```python
from build123d import *

# Parameters (mm, degrees)
SKETCH1_W           = 25.5
SKETCH1_H           = 5.5
BOSS_EXTRUDE1_DEPTH = 5
CUT_EXTRUDE1_DEPTH  = 10
SKETCH5_W           = 60
SKETCH5_H           = 5
BOSS_EXTRUDE2_DEPTH = 5
SKETCH6_W           = 20.4
SKETCH6_H           = 5
CUT_EXTRUDE2_DEPTH  = 10


with BuildPart() as part:
    # Sketch1 → Boss-Extrude1 (new body)
    with BuildSketch(Plane.XY):
        Polygon((-155, 151.5), (-155, 146.5), (5, 146.5), (5, 151.5), (25, 151.5), (25, -8.5), (-170, -8.5), (-170, 17.5), (-150, 17.5), (-150, 22.5), (-170, 22.5), (-170, 41), (-170, 41.4), (-163.2, 41.4), (-163.2, 40), (-160, 40), (-160, 41.4), (-153, 41.4), (-153, 45.6), (-160, 45.6), (-160, 47), (-163.2, 47), (-163.2, 45.6), (-170, 45.6), (-170, 46), (-170, 64.5), (-150, 64.5), (-150, 69.5), (-170, 69.5), (-170, 88.4), (-163.2, 88.4), (-163.2, 87), (-160, 87), (-160, 88.4), (-153, 88.4), (-153, 92.6), (-160, 92.6), (-160, 94), (-163.2, 94), (-163.2, 92.6), (-170, 92.6), (-170, 111.5), (-150, 111.5), (-150, 116.5), (-170, 116.5), (-170, 146.5), (-175, 146.5), (-175, 151.5), align=None)
        with Locations((-58.25, 13.75)):
            Rectangle(SKETCH1_W, SKETCH1_H, mode=Mode.SUBTRACT)
        with Locations((-12.75, 2.75)):
            Rectangle(SKETCH1_W, SKETCH1_H, mode=Mode.SUBTRACT)
        with Locations((-58.25, 2.75)):
            Rectangle(SKETCH1_W, SKETCH1_H, mode=Mode.SUBTRACT)
        with Locations((-12.75, 13.75)):
            Rectangle(SKETCH1_W, SKETCH1_H, mode=Mode.SUBTRACT)
        with Locations((-12.75, 26.25)):
            Rectangle(SKETCH1_W, SKETCH1_H, mode=Mode.SUBTRACT)
        with Locations((-58.25, 26.25)):
            Rectangle(SKETCH1_W, SKETCH1_H, mode=Mode.SUBTRACT)
        with Locations((-58.25, 37.25)):
            Rectangle(SKETCH1_W, SKETCH1_H, mode=Mode.SUBTRACT)
        with Locations((-12.75, 37.25)):
            Rectangle(SKETCH1_W, SKETCH1_H, mode=Mode.SUBTRACT)
        with Locations((-12.75, 49.75)):
            Rectangle(SKETCH1_W, SKETCH1_H, mode=Mode.SUBTRACT)
        with Locations((-58.25, 49.75)):
            Rectangle(SKETCH1_W, SKETCH1_H, mode=Mode.SUBTRACT)
        with Locations((-58.25, 60.75)):
            Rectangle(SKETCH1_W, SKETCH1_H, mode=Mode.SUBTRACT)
        with Locations((-12.75, 60.75)):
            Rectangle(SKETCH1_W, SKETCH1_H, mode=Mode.SUBTRACT)
        with Locations((-12.75, 73.25)):
            Rectangle(SKETCH1_W, SKETCH1_H, mode=Mode.SUBTRACT)
        with Locations((-58.25, 73.25)):
            Rectangle(SKETCH1_W, SKETCH1_H, mode=Mode.SUBTRACT)
        with Locations((-58.25, 84.25)):
            Rectangle(SKETCH1_W, SKETCH1_H, mode=Mode.SUBTRACT)
        with Locations((-12.75, 84.25)):
            Rectangle(SKETCH1_W, SKETCH1_H, mode=Mode.SUBTRACT)
        with Locations((-12.75, 96.75)):
            Rectangle(SKETCH1_W, SKETCH1_H, mode=Mode.SUBTRACT)
        with Locations((-58.25, 96.75)):
            Rectangle(SKETCH1_W, SKETCH1_H, mode=Mode.SUBTRACT)
        with Locations((-58.25, 107.75)):
            Rectangle(SKETCH1_W, SKETCH1_H, mode=Mode.SUBTRACT)
        with Locations((-12.75, 107.75)):
            Rectangle(SKETCH1_W, SKETCH1_H, mode=Mode.SUBTRACT)
        with Locations((-12.75, 120.25)):
            Rectangle(SKETCH1_W, SKETCH1_H, mode=Mode.SUBTRACT)
        with Locations((-58.25, 120.25)):
            Rectangle(SKETCH1_W, SKETCH1_H, mode=Mode.SUBTRACT)
        with Locations((-58.25, 131.25)):
            Rectangle(SKETCH1_W, SKETCH1_H, mode=Mode.SUBTRACT)
        with Locations((-12.75, 131.25)):
            Rectangle(SKETCH1_W, SKETCH1_H, mode=Mode.SUBTRACT)
    extrude(amount=BOSS_EXTRUDE1_DEPTH)

    # Sketch4 → Cut-Extrude1 (cut)
    with BuildSketch(Plane.XY.offset(5)):
        Polygon((-37.8, 129.5), (-37.8, 136.5), (-39.2, 136.5), (-39.2, 139.7), (-37.8, 139.7), (-37.8, 146.5), (-33.6, 146.5), (-33.6, 139.7), (-32.2, 139.7), (-32.2, 136.5), (-33.6, 136.5), (-33.6, 129.5), align=None)
        Polygon((-139.2, 139.7), (-139.2, 146.5), (-135, 146.5), (-135, 139.7), (-133.6, 139.7), (-133.6, 136.5), (-135, 136.5), (-135, 129.5), (-139.2, 129.5), (-139.2, 136.5), (-140.6, 136.5), (-140.6, 139.7), align=None)
        Polygon((-37.8, -8.5), (-33.6, -8.5), (-33.6, -1.7), (-32.2, -1.7), (-32.2, 1.5), (-33.6, 1.5), (-33.6, 8.5), (-37.8, 8.5), (-37.8, 1.5), (-39.2, 1.5), (-39.2, -1.7), (-37.8, -1.7), align=None)
        Polygon((-139.2, -8.5), (-135, -8.5), (-135, -1.7), (-133.6, -1.7), (-133.6, 1.5), (-135, 1.5), (-135, 8.5), (-139.2, 8.5), (-139.2, 1.5), (-140.6, 1.5), (-140.6, -1.7), (-139.2, -1.7), align=None)
    extrude(amount=-CUT_EXTRUDE1_DEPTH, mode=Mode.SUBTRACT)

    # Sketch5 → Boss-Extrude2 (add)
    with BuildSketch(Plane(origin=(0, 0, 0), x_dir=(-1, 0, 0), z_dir=(0, 0, -1))):
        with Locations((80, -11)):
            Rectangle(SKETCH5_W, SKETCH5_H)
    extrude(amount=-BOSS_EXTRUDE2_DEPTH)

    # Sketch6 → Cut-Extrude2 (cut)
    with BuildSketch(Plane(origin=(0, 0, 0), x_dir=(-1, 0, 0), z_dir=(0, 0, -1))):
        with Locations((159.8, 114)):
            Rectangle(SKETCH6_W, SKETCH6_H)
        with Locations((159.8, 67)):
            Rectangle(SKETCH6_W, SKETCH6_H)
        with Locations((159.8, 20)):
            Rectangle(SKETCH6_W, SKETCH6_H)
    extrude(amount=-CUT_EXTRUDE2_DEPTH, mode=Mode.SUBTRACT)


solid = part.part
```
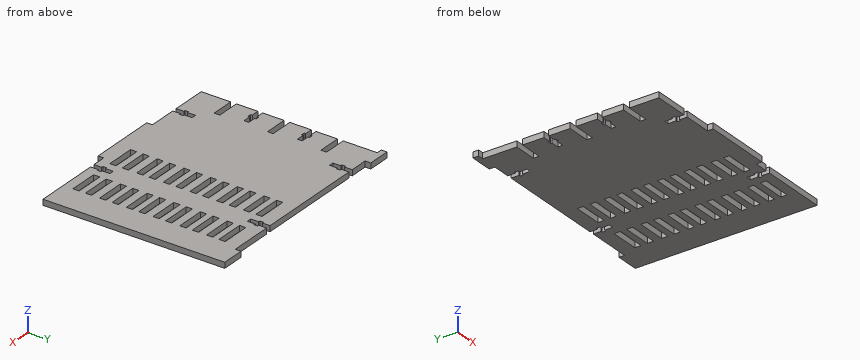
Here's how the part is built. I have some questions about the finished solid (model axes, mm). Round coordinates to 2 decimals unless told otherwise and drop trailing zeros. Write each loop counter-clockwise with the first axis right and the second up, starting at its lowest first coordinate (ties: lowest second). Pieces come first, ordered by that corner, then holes.
Q1. Will these pins go through, and if not, where does the flat tip stop? P1, Ø1.5, axis at x = -161.5, z = 2.5, coming from the -Y side; P2, Ø2, axis at y = 42.5, z = 2, coming from the -X side; P3, Ø1.5, axis at y = 1.5, z = 3, coming from the -X side.
Q2. If we section it at B-B on x = -66.5: Give the number of separate pieces and of enclosed holes in the cut face, plus the area to 3 significant figures.
Q3. If we section it at A-A on y = 97: Write out the boundary of the cut face in (x, z).
Q4. Please list where these lines run through material, in increasing order: probe 1 along X at (y, z) = (109, 0.7); probe 2 along X at (y, z) = (7, 1.7); probe 3 along Y at (x, z) = (-145, 1.3).
Q5. If we section it at D-D on x = -91: Write out the boundary of the cut face in (y, z), plus the area to 3 significant figures.
Answer below:
1. P1: stops at y = -8.5
1. P2: stops at x = -153
1. P3: stops at x = -170
2. separate pieces: 13
2. enclosed holes: 0
2. area: 470 mm2
3. outline: (-170, 0) - (-71, 0) - (-71, 5) - (-170, 5) - close; (-45.5, 0) - (-25.5, 0) - (-25.5, 5) - (-45.5, 5) - close; (0, 0) - (25, 0) - (25, 5) - (0, 5) - close
4. probe 1: x = -170 to -71, -45.5 to -25.5, 0 to 25
4. probe 2: x = -170 to -139.2, -135 to -37.8, -33.6 to 25
4. probe 3: y = -8.5 to 146.5
5. outline: (-13.5, 0) - (146.5, 0) - (146.5, 5) - (-13.5, 5) - close
5. area: 800 mm2
